Could you check a few things on this model? Use its own coordinates, in mm. A direction names the side the tool comes from. Coordinates: 2 decimals unless noted, no trailing zeros. Write each loop counter-clockwise with the first axis right and the second up, starting at its lowest first coordinate (ties: lowest second). Pieces come first, ordered by that corner, then holes. Notation, with made-up numbers: M -25.75,55 L 7.25,55 A25 cw 7.25,70 Z; hole C 20,26 d10. An arc over 180 degrees is marked long. Write item = value, one per line.
```python
from build123d import *

# Parameters (mm, degrees)
CROQUIS1_R              = 1.5
CROQUIS1_R_2            = 3.6
SALIENTE_EXTRUIR2_DEPTH = 9


with BuildPart() as part:
    # Croquis1 → Saliente-Extruir2 (new body)
    with BuildSketch(Plane(origin=(0, 0, 0), x_dir=(1, 0, 0), z_dir=(0, 1, 0))):
        Polygon((7.75, 7.5), (26.5, 22.904273087), (26.5, 77.904273087), (26.5, 87.904273087), (41.5, 77.904273087), (41.5, 22.904273087), (22.75, 7.5), (22.75, -7.5), (7.75, -7.5), align=None)
        with Locations(Location((19.25, 4, 0), (0, 0, 270))):
            Circle(CROQUIS1_R, mode=Mode.SUBTRACT)
        with Locations(Location((19.25, -4, 0), (0, 0, 270))):
            Circle(CROQUIS1_R, mode=Mode.SUBTRACT)
        with Locations(Location((11.25, -4, 0), (0, 0, 270))):
            Circle(CROQUIS1_R, mode=Mode.SUBTRACT)
        with Locations(Location((11.25, 4, 0), (0, 0, 270))):
            Circle(CROQUIS1_R, mode=Mode.SUBTRACT)
        with Locations(Location((15.25, 0, 0), (0, 0, 270))):
            Circle(CROQUIS1_R_2, mode=Mode.SUBTRACT)
    extrude(amount=SALIENTE_EXTRUIR2_DEPTH)


solid = part.part
```
Item 1: Imagine slicing it at D-D (z = -68). Write out the boundary of the cut face in (x, y), and give its area (3 significant figures).
Numbers:
outline = M 26.5,0 L 41.5,0 L 41.5,9 L 26.5,9 Z
area = 135 mm²
Item 2: Imagine slicing it at C-C (x = 15.25). Write out the boundary of the cut face in (y, z).
Numbers:
outline = M 0,-13.66 L 9,-13.66 L 9,-3.6 L 0,-3.6 Z; M 0,3.6 L 9,3.6 L 9,7.5 L 0,7.5 Z
Item 3: If we mould it in two halves opening along X, with no side actions, what happens to faces 4 (the face through (11.7, 4.44, -2.57)), 5 (the face through (32.256, 4.437, -15.31)), 6 (the face through (29, 0, -41))? For each: pulls with the +X half, pulls with the -X half, needs draft (parallel to the pull), parting line crosses it, or undercut.
Numbers:
face_4 = undercut
face_5 = pulls with the +X half
face_6 = needs draft
Item 4: If I drill on line 1 along X through (y, z) = (4.5, -41.5); line 2 along X through (y, z) = (2, 2); line 3 along Z through (x, y) = (28.5, 5.25), over which ranges is the centre line in solid material (lowest first)?
Numbers:
line_1 = 26.5 to 41.5
line_2 = 7.75 to 12.26, 18.24 to 22.75
line_3 = -86.57 to -12.22
Item 5: Imagine slicing it at B-B (y = 4.25). Write out the boundary of the cut face in (x, z), and give its area (3 significant figures).
Numbers:
outline = M 7.75,-7.5 L 26.5,-22.9 L 26.5,-87.9 L 41.5,-77.9 L 41.5,-22.9 L 22.75,-7.5 L 22.75,7.5 L 7.75,7.5 Z; hole C 11.25,-4 d3; hole C 11.25,4 d3; hole C 15.25,0 d7.2; hole C 19.25,-4 d3; hole C 19.25,4 d3
area = 1,290 mm²
Item 6: Imagine slicing it at A-A (z = 0). Write out the boundary of the cut face in (x, y), and give its area (3 significant figures).
Numbers:
outline = M 7.75,0 L 11.65,0 L 11.65,9 L 7.75,9 Z; M 18.85,0 L 22.75,0 L 22.75,9 L 18.85,9 Z
area = 70.2 mm²
Item 7: For faces 1 (the face through (33.9, 4.44, -82.97)), 2 (the face through (26.5, 4, -56)), 3 (the face through (22.75, 4, 0)), which set-ups out of +Z, -Z, +X, -X, +Y, -Y let a thin tool reach every point of the face, with its end or its side?
Numbers:
face_1 = -Z, +X, +Y, -Y
face_2 = -Z, -X, +Y, -Y
face_3 = +Z, +X, +Y, -Y
Item 8: I'm going to push flat-ended pins straight in: P1, Ø4, axis at x = 32.5, z = -64, coming from the -Y side; P2, Ø2.5, axis at x = 19.25, z = -4, coming from the -Y side; P3, Ø5, axis at y = 5, z = -4, coming from the +X side; P4, Ø2, axis at y = 6, z = -10, coming from the -X side. Where does each tip first touch, or does it pass through?
Numbers:
P1 = 0
P2 = through
P3 = 22.75
P4 = 9.58
